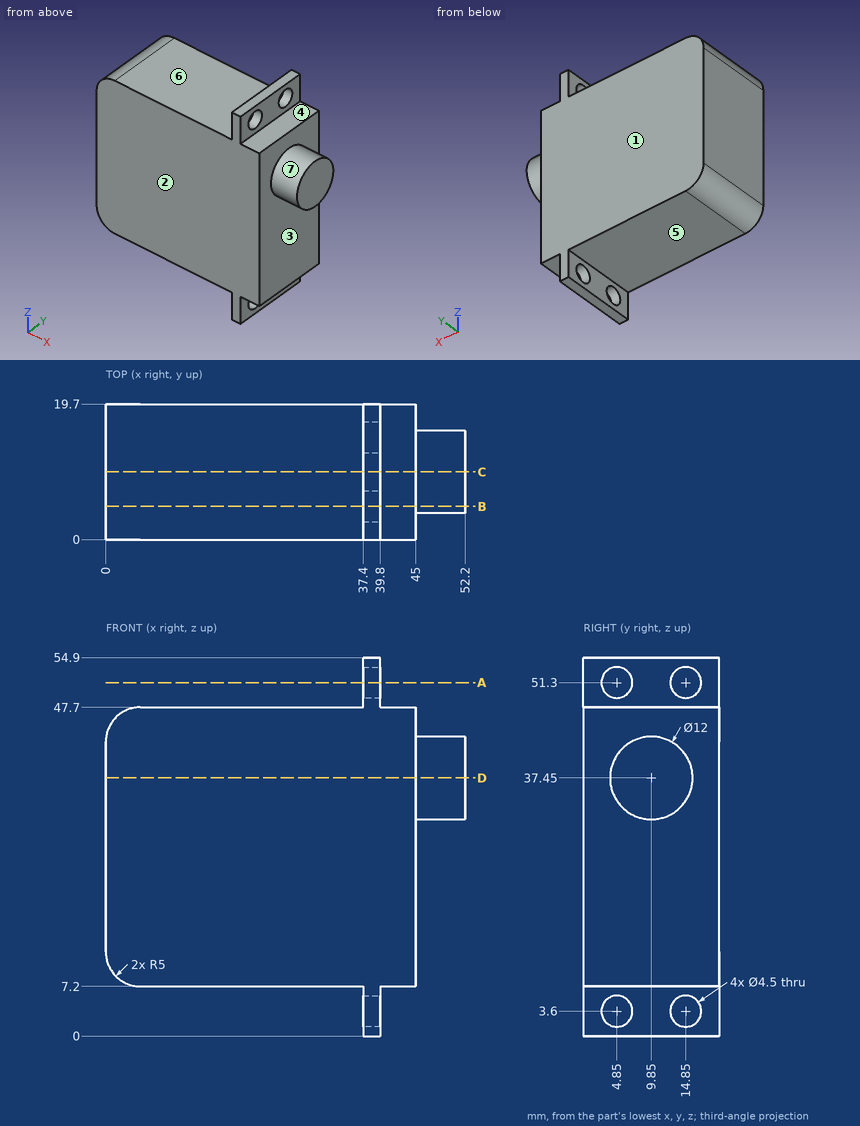
Print and shaded views of the part. All mm, measured from the part's lowest x, y and z. A direction names the side the tool comes from. Round coordinates to 2 decimals unless told otherwise and drop trailing zeros. Write each loop counter-clockwise with the first axis right and the second up, starting at its lowest first coordinate (ties: lowest second). Pieces come first, ordered by that corner, then holes.
(1) 3-axis set-ups, long thin cutter, end or side, ignore diameter. For the marked faces 4, 5, 6 and 7: which of +Z, -Z, +X, -X, +Y, -Y reach the whole face in a straight line?
(2) Drop flat-ended pins along their axis: P1, Ø6, axis at y = 14, z = 19.5, coming from the +X side; P2, Ø7, axis at y = 14.85, z = 51.3, coming from the +X side; P3, Ø2.5, axis at x = 41.5, y = 10.5, coming from the -Z side. Give the stop position or say it passes through.
(3) Slice it at D-D, the plane z = 37.45. Write the cut outline in (x, y).
(4) Slice it at A-A, the plane z = 51.3. Write the cut outline in (x, y).
(5) Slice it at C-C, the plane y = 9.85. Write the cut outline in (x, z), and give its area (3 significant figures).
(6) Probe line 1 along Y through (x, z) = (38, 51.3); line 2 along Z through (x, y) = (17, 17.5); line 3 along Y through (x, z) = (38, 3). List the from-to ranges inside material, lowest first.
(7) Mould opens along Y. For the marked faces 1, 2 and 3 say: pulls with the +Y half, pulls with the -Y half, needs draft (parallel to the pull), parting line crosses it, or undercut.
(8) Slice it at B-B, the plane y = 4.85. Write the cut outline in (x, z).
From the geometry:
1. face 4: +Z, +X, +Y, -Y
1. face 5: -Z, -X, +Y, -Y
1. face 6: +Z, -X, +Y, -Y
1. face 7: +X
2. P1: stops at x = 45
2. P2: stops at x = 39.8
2. P3: stops at z = 7.2
3. outline: (0, 0) - (45, 0) - (45, 3.85) - (52.2, 3.85) - (52.2, 15.85) - (45, 15.85) - (45, 19.7) - (0, 19.7) - close
4. outline: (37.4, 0) - (39.8, 0) - (39.8, 2.6) - (37.4, 2.6) - close; (37.4, 7.1) - (39.8, 7.1) - (39.8, 12.6) - (37.4, 12.6) - close; (37.4, 17.1) - (39.8, 17.1) - (39.8, 19.7) - (37.4, 19.7) - close
5. outline: (0, 12.2) arc R5 ccw to (5, 7.2) - (37.4, 7.2) - (37.4, 0) - (39.8, 0) - (39.8, 7.2) - (45, 7.2) - (45, 31.45) - (52.2, 31.45) - (52.2, 43.45) - (45, 43.45) - (45, 47.7) - (39.8, 47.7) - (39.8, 54.9) - (37.4, 54.9) - (37.4, 47.7) - (5, 47.7) arc R5 ccw to (0, 42.7) - close
5. area: 1,930 mm2
6. line 1: y = 0 to 2.6, 7.1 to 12.6, 17.1 to 19.7
6. line 2: z = 7.2 to 47.7
6. line 3: y = 0 to 2.68, 7.02 to 12.68, 17.02 to 19.7
7. face 1: pulls with the +Y half
7. face 2: pulls with the -Y half
7. face 3: needs draft
8. outline: (0, 12.2) arc R5 ccw to (5, 7.2) - (37.4, 7.2) - (37.4, 5.85) - (39.8, 5.85) - (39.8, 7.2) - (45, 7.2) - (45, 34.13) - (52.2, 34.13) - (52.2, 40.77) - (45, 40.77) - (45, 47.7) - (39.8, 47.7) - (39.8, 49.05) - (37.4, 49.05) - (37.4, 47.7) - (5, 47.7) arc R5 ccw to (0, 42.7) - close; (37.4, 0) - (39.8, 0) - (39.8, 1.35) - (37.4, 1.35) - close; (37.4, 53.55) - (39.8, 53.55) - (39.8, 54.9) - (37.4, 54.9) - close
